```python
from build123d import *

# Parameters (mm, degrees)
F0_W      = 75
F0_H      = 65
F1_DEPTH  = 8
F2_R      = 2
F3_W      = 68.330624
F3_H      = 51.542157
F4_DEPTH  = 8.001
F5_W      = 0.7
F5_H      = 7.5
F6_DEPTH  = 4
F7_R      = 1.3
F9_DEPTH  = 5
F8_R      = 1.3
F10_DEPTH = 5


with BuildPart() as f1:
    # F0 (on Top) → F1 (new body)
    with BuildSketch(Plane.XY):
        Rectangle(F0_W, F0_H)
    extrude(amount=F1_DEPTH)

    # F2
    f2_edges = [f1.edges().sort_by_distance(p)[0] for p in [
        (0, -32.5, 8),
        (37.5, 0, 8),
        (0, 32.5, 8),
        (-37.5, 0, 8),
    ]]
    fillet(f2_edges, radius=F2_R)

    # F3 (on face) → F4 (cut, through all)
    with BuildSketch(Plane.XY.offset(8)):
        with Locations((0.502158, 0.043064)):
            Rectangle(F3_W, F3_H)
    extrude(amount=-F4_DEPTH, mode=Mode.SUBTRACT)

    # F5 (on face) → F6 (cut)
    with BuildSketch(Plane.XY.offset(8)):
        with Locations((-28.739675, 27.984681)):
            Rectangle(F5_W, F5_H)
        with Locations((-28.739675, -29.515319)):
            Rectangle(F5_W, F5_H)
        with Locations((-19.939675, 27.984681)):
            Rectangle(F5_W, F5_H)
        with Locations((-19.939675, -29.515319)):
            Rectangle(F5_W, F5_H)
        with Locations((-11.139675, 27.984681)):
            Rectangle(F5_W, F5_H)
        with Locations((-11.139675, -29.515319)):
            Rectangle(F5_W, F5_H)
        with Locations((-2.339675, 27.984681)):
            Rectangle(F5_W, F5_H)
        with Locations((-2.339675, -29.515319)):
            Rectangle(F5_W, F5_H)
        with Locations((6.460325, 27.984681)):
            Rectangle(F5_W, F5_H)
        with Locations((6.460325, -29.515319)):
            Rectangle(F5_W, F5_H)
        with Locations((15.260325, 27.984681)):
            Rectangle(F5_W, F5_H)
        with Locations((15.260325, -29.515319)):
            Rectangle(F5_W, F5_H)
        with Locations((24.060325, 27.984681)):
            Rectangle(F5_W, F5_H)
        with Locations((24.060325, -29.515319)):
            Rectangle(F5_W, F5_H)
        with Locations((32.860325, 27.984681)):
            Rectangle(F5_W, F5_H)
        with Locations((32.860325, -29.515319)):
            Rectangle(F5_W, F5_H)
    extrude(amount=-F6_DEPTH, mode=Mode.SUBTRACT)

    # F7 (on face) → F9 (cut)
    with BuildSketch(Plane.XZ.offset(32.5)):
        with Locations((-32.797666, 3.178249)):
            Circle(F7_R)
        with Locations((28.105985, 3.178249)):
            Circle(F7_R)
    extrude(amount=-F9_DEPTH, mode=Mode.SUBTRACT)

    # F8 (on face) → F10 (cut)
    with BuildSketch(Plane(origin=(0, 32.5, 0), x_dir=(-1, 0, 0), z_dir=(0, 1, 0))):
        with Locations((32.797666, 3.178249)):
            Circle(F8_R)
        with Locations((-28.105985, 3.178249)):
            Circle(F8_R)
    extrude(amount=-F10_DEPTH, mode=Mode.SUBTRACT)


solid = f1.part
```
The model under review builds one solid part; all positions refer to its coordinate system, in mm. A direction names the side the tool comes from. Give positions to 0.01 mm unless a question says otherwise; leave off trailing zeros. Write each loop counter-clockwise with the first axis right and the second up, starting at its lowest first coordinate (ties: lowest second). Pieces come first, ordered by that corner, then holes.
(1) Consider section A-A, the plane y = -10.5. Give the boundary of the cut face in (x, z), and give its area (3 significant figures).
(2) Tool access review of faces 1 (the flat face through (-2.69, 29, 6)), 2 (the cylindrical face through (27.07, -30.04, 2.39)), 3 (the flat face through (-11.49, -29, 6)): name each direction out of +Z, -Z, +X, -X, +Y, -Y from which nothing blocks a thin tool from reaching the whole face with its end or side.
(3) The part is to be moulded in two halves that separate along Y. For faces 4 (the flat face through (33.21, 29, 6)), 5 (the flat face through (-20.29, -29, 6)), 6 (the flat face through (-33, -27.5, 3)), say which applies: released by +Y, released by -Y, zero draft, split by the parting line, or undercut.
(4) To check wall thickness, follow L1, parallel to Y at x = 5, z = 1.5; L2, parallel to X at y = 21.5, z = 5.5; L3, parallel to Y at x = -13.5, z = 7. State the ranges of each line that lie inside material, in increasing order.
(5) Consider section B-B, the plane x = 31. Give the boundary of the cut face in (y, z).
(6) For P1, Ø2, axis at x = 1, y = 25.5, coming from the +Z side; P2, Ø1.6, axis at x = -32.8, z = 3.18, coming from the +Y side; P3, Ø1.3, axis at x = -33, z = 3.5, coming from the -Y side, all flat-tipped, find the tip position at first contact; note any pin that passes through.
Returned:
1. outline: (-37.5, 0) - (-33.66, 0) - (-33.66, 8) - (-35.5, 8) arc R2 ccw to (-37.5, 6) - close; (34.67, 0) - (37.5, 0) - (37.5, 6) arc R2 ccw to (35.5, 8) - (34.67, 8) - close
1. area: 51.6 mm2
2. face 1: +Z
2. face 2: -Y
2. face 3: +Z, -Y
3. face 4: undercut
3. face 5: zero draft
3. face 6: released by -Y
4. L1: y = -32.5 to -25.73, 25.81 to 32.5
4. L2: x = -37.5 to -33.66, 34.67 to 37.5
4. L3: y = -32.23 to -25.73, 25.81 to 32.23
5. outline: (-32.5, 0) - (-25.73, 0) - (-25.73, 8) - (-30.5, 8) arc R2 ccw to (-32.5, 6) - close; (25.81, 0) - (32.5, 0) - (32.5, 6) arc R2 ccw to (30.5, 8) - (25.81, 8) - close
6. P1: stops at z = 8
6. P2: stops at y = 27.5
6. P3: stops at y = -27.5
